Check sheet for the modelled part. Datum: model origin and axes. Units: mm. A direction names the side the tool comes from. Coordinates: 2 decimals unless noted, no trailing zeros. Write each loop counter-clockwise with the first axis right and the second up, starting at its lowest first coordinate (ties: lowest second). Pieces come first, ordered by that corner, then holes. Notation, with made-up numbers: M -12.5,63.5 L -1.5,63.5 A15 cw -1.5,72.5 Z; hole C -35,9.5 d4. An arc over 180 degrees is marked long. Answer as CSV lines item,"result". Start each with the question number.
Q1. Thickness scan on line 1 along Z through (x, y) = (169, -0.5); line 2 along Y through (x, z) = (343, -8.5); line 3 along Z through (x, y) = (192.5, -4). Record the ranges inside material, lowest first. Write a range as from..to.
Q2. Sectioned sample at B-B, the plane z = 0. Record the cut outline in (x, y), then the cut area to 3 significant figures.
Q3. Sectioned sample at A-A, the plane x = 256. Record the cut outline in (y, z).
Q4. Access from +Z, -Z, +X, -X, +Y, -Y to the whole of each face (thin tool, end or side, straight path). Record for faces 1 (the cylindrical face through (170.246, 4.213, 10.161)), 2 (the flat face through (-53, 0, 0)).
Q5. Depth check by flat-ended pin: pin 1 Ø6 at (y, z) = (-23, 12) entering from +X; pin 2 Ø5 at (x, y) = (56, -7) entering from +Z; pin 3 Ø5 at (y, z) = (26.5, 22) entering from -X. Enter the tip coordinate at first touch or a pass-through.
from build123d import *

# Parameters (mm, degrees)
CHAMFER1_SIZE = 1


with BuildPart() as part:
    # Sketch1 → Revolve1 (revolve)
    with BuildSketch(Plane.XY, mode=Mode.PRIVATE) as revolve1_sk:
        Polygon((-39, 8.5), (-39, 5.6), (-53, 5.6), (-53, 0), (411.5, 0), (411.5, 11), (0, 11), (0, 8.5), align=None)
    revolve(revolve1_sk.sketch.rotate(Axis((-53, 0, 0), (1, 0, 0)), 90), axis=Axis((-53, 0, 0), (1, 0, 0)))

    # Chamfer1
    chamfer1_edges = [part.edges().sort_by_distance(p)[0] for p in [
        (-53, 0, -5.6),
    ]]
    chamfer(chamfer1_edges, length=CHAMFER1_SIZE)

    # Sketch2 → Revolve2 (revolve)
    with BuildSketch(Plane(origin=(0, 0, 0), x_dir=(1, 0, 0), z_dir=(0, 1, 0))):
        with BuildLine():
            Line((371.5, 0), (451.5, 0))
            ThreePointArc((451.5, 0), (411.5, 40), (371.5, 0))
        make_face()
    revolve(axis=Axis((371.5, 0, 0), (1, 0, 0)))

    # Fillet1: read off the stored shape, not the designer's step
    # Fillet1 outline → Fillet1 (revolve)
    with BuildSketch(Plane.YX):
        with BuildLine():
            ThreePointArc((11, 345.325986974), (15.20456112, 365.395311272), (27.111111111, 382.089327544))
            Line((27.111111111, 382.089327544), (11, 382.089327544))
            Line((11, 382.089327544), (11, 345.325986974))
        make_face()
    revolve(axis=Axis((0, 0, 0), (1, 0, 0)))

    # Sketch3 → Cut-Revolve1 (revolve, cut)
    with BuildSketch(Plane(origin=(0, 0, 0), x_dir=(1, 0, 0), z_dir=(0, 1, 0))):
        with BuildLine():
            Line((426.5, 0), (451.5, 0))
            ThreePointArc((451.5, 0), (444.666247904, 22.360679775), (426.5, 37.080992435))
            Line((426.5, 37.080992435), (426.5, 0))
        make_face()
    revolve(axis=Axis((426.5, 0, 0), (1, 0, 0)), mode=Mode.SUBTRACT)

    # Sketch4 → Cut-Revolve2 (revolve, cut)
    with BuildSketch(Plane(origin=(0, 0, 0), x_dir=(1, 0, 0), z_dir=(0, 1, 0))):
        with BuildLine():
            Line((376.5, 0), (446.5, 0))
            ThreePointArc((446.5, 0), (411.5, 35), (376.5, 0))
        make_face()
    revolve(axis=Axis((376.5, 0, 0), (1, 0, 0)), mode=Mode.SUBTRACT)


solid = part.part
Output:
1,line 1,"z = -10.99..10.99"
1,line 2,"y = -6.98..6.98"
1,line 3,"z = -10.25..10.25"
2,outline,"M -53,-4.6 L -52,-5.6 L -39,-5.6 L -39,-8.5 L 0,-8.5 L 0,-11 L 345.33,-11 A50 cw 382.09,-27.11 A40 ccw 426.5,-37.08 L 426.5,-31.62 A35 cw long 426.5,31.62 L 426.5,37.08 A40 ccw 382.09,27.11 A50 cw 345.33,11 L 0,11 L 0,8.5 L -39,8.5 L -39,5.6 L -52,5.6 L -53,4.6 Z"
2,area,"9,940 mm^2"
3,outline,"C 0,0 d22"
4,face 1,"-X"
4,face 2,"+Z, -Z, -X, +Y, -Y"
5,pin 1,"stops at x = 391.82"
5,pin 2,"stops at z = 10.04"
5,pin 3,"stops at x = 387.42"
